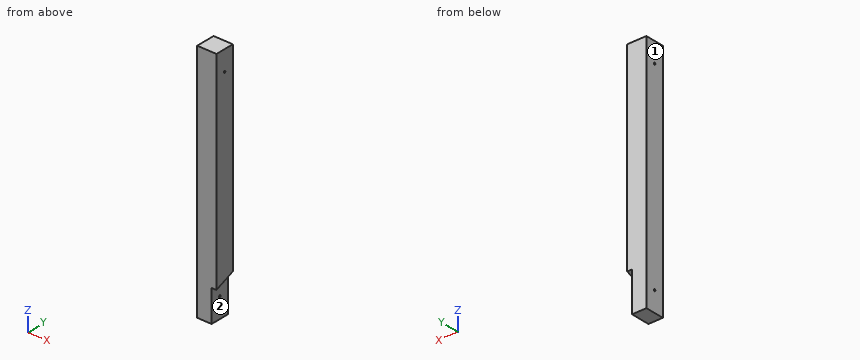
```python
from build123d import *

# Parameters (mm, degrees)
SKETCH1_W           = 100
SKETCH1_H           = 100
BOSS_EXTRUDE1_DEPTH = 625
SKETCH2_R           = 5
CUT_EXTRUDE1_DEPTH  = 635.92125496
CUT_EXTRUDE2_DEPTH  = 25


with BuildPart() as part:
    # Sketch1 → Boss-Extrude1 (new, symmetric)
    with BuildSketch(Plane.XY):
        Rectangle(SKETCH1_W, SKETCH1_H)
    extrude(amount=BOSS_EXTRUDE1_DEPTH, both=True)

    # Sketch2 → Cut-Extrude1 (cut, through all)
    with BuildSketch(Plane.ZY.offset(50)):
        with Locations(Location((-520, 0, 0), (0, 0, 270))):
            Circle(SKETCH2_R)
        with Locations(Location((520, 0, 0), (0, 0, 270))):
            Circle(SKETCH2_R)
    extrude(amount=-CUT_EXTRUDE1_DEPTH, mode=Mode.SUBTRACT)

    # Sketch3 → Cut-Extrude2 (cut)
    with BuildSketch(Plane(origin=(50, 0, 0), x_dir=(0, 0, -1), z_dir=(1, 0, 0))):
        Polygon((418.892046252, 50), (459.315842164, -50), (625, -50), (625, 50), align=None)
    extrude(amount=-CUT_EXTRUDE2_DEPTH, mode=Mode.SUBTRACT)


solid = part.part
```
Geometry check sheet. Reference: the model listing, model coordinates, mm. Face numbers are marked on the shaded views. A direction names the side the tool comes from. Round coordinates to 2 decimals unless told otherwise and drop trailing zeros. Order: outer loops, then holes, each group sorted by start corner. A loop starts at its lowest first (then second) coordinate and runs counter-clockwise, first axis right, second up. Notation, with made-up numbers: (50, 36) -> (73, 36) arc R19 cw to (73, 56) -> close; hole circle Ø8 at (30, 62.25). An arc over 180 degrees is marked (long way). Return JSON: item names as keys, results as strings. Group by question number.
Q1. Gauge pin test, flat ends, axial feed: pin 1 (11.5 mm diameter, centred on y = 0, z = -520, fed in from +X); pin 2 (8 mm diameter, centred on y = 0, z = 520, fed in from -X). Record the tip position at first contact, or that the pin passes through.
Q2. Section check A-A, the plane y = -32. Record the boundary of the cut face in (x, z), plus the area to 3 significant figures.
Q3. Material ranges on probe 1 along Z at (x, y) = (6, 0); probe 2 along Z at (x, y) = (-12, -1.5); probe 3 along Y at (x, z) = (1.5, -520), recorded low to high. Write a range as from..to.
Q4. Tool access check on the marked faces 1 and 2. Record the directions out of +Z, -Z, +X, -X, +Y, -Y that give a thin tool (end or side, any length) a straight path to the whole face; none if there is none.
Q5. Section check B-B, the plane y = 32. Record the boundary of the cut face in (x, z).
Numbers:
{
 "1": {"pin 1": "x = 25", "pin 2": "through"},
 "2": {"outline": "(-50, -625) -> (25, -625) -> (25, -452.04) -> (50, -452.04) -> (50, 625) -> (-50, 625) -> close", "area": "121,000 mm^2"},
 "3": {"probe 1": "-625..-525, -515..515, 525..625", "probe 2": "-625..-524.77, -515.23..515.23, 524.77..625", "probe 3": "-50..-5, 5..50"},
 "4": {"face 1": "+Z, -Z, -X, +Y, -Y", "face 2": "-Z, +X, +Y"},
 "5": {"outline": "(-50, -625) -> (25, -625) -> (25, -426.17) -> (50, -426.17) -> (50, 625) -> (-50, 625) -> close"}
}
